CAD build for the part. Positions are in the model's coordinates, mm. Face numbers are marked on the shaded views. A direction names the side the tool comes from. Coordinates: 2 decimals unless noted, no trailing zeros. Order: outer loops, then holes, each group sorted by start corner. A loop starts at its lowest first (then second) coordinate and runs counter-clockwise, first axis right, second up. Notation, with made-up numbers: (88.5, 54) - (118.5, 54) arc R12 cw to (118.5, 63) - close; hole circle Ø7 at (-14.75, 31). An arc over 180 degrees is marked (long way). Use one line per item in the form item = value.
```python
from build123d import *

# Parameters (mm, degrees)
F0_R      = 8.89
F1_DEPTH  = 17.78
F2_R      = 7.747
F3_DEPTH  = 38.989
F4_R      = 8.89
F5_DEPTH  = 1.905
F6_R      = 7.747
F7_DEPTH  = 2.032
F8_R      = 8.89
F9_DEPTH  = 13.335
F10_R     = 7.747
F11_DEPTH = 2.032
F12_R     = 8.89
F13_DEPTH = 1.905
F14_R     = 7.747
F15_DEPTH = 12.7
F16_R     = 8.89
F17_DEPTH = 28.575
F18_R     = 6.477
F19_DEPTH = 27.559


with BuildPart() as f1:
    # F0 (on Right) → F1 (new body)
    with BuildSketch(Plane.YZ):
        Circle(F0_R)
    extrude(amount=F1_DEPTH)

    # F2 (on face) → F3 (join)
    with BuildSketch(Plane.YZ.offset(17.78)):
        Circle(F2_R)
    extrude(amount=F3_DEPTH)

    # F4 (on face) → F5 (join)
    with BuildSketch(Plane.YZ.offset(56.769)):
        Circle(F4_R)
    extrude(amount=F5_DEPTH)

    # F6 (on face) → F7 (join)
    with BuildSketch(Plane.YZ.offset(58.674)):
        Circle(F6_R)
    extrude(amount=F7_DEPTH)

    # F8 (on face) → F9 (join)
    with BuildSketch(Plane.YZ.offset(60.706)):
        Circle(F8_R)
    extrude(amount=F9_DEPTH)

    # F10 (on face) → F11 (join)
    with BuildSketch(Plane.YZ.offset(74.041)):
        Circle(F10_R)
    extrude(amount=F11_DEPTH)

    # F12 (on face) → F13 (join)
    with BuildSketch(Plane.YZ.offset(76.073)):
        Circle(F12_R)
    extrude(amount=F13_DEPTH)

    # F14 (on face) → F15 (join)
    with BuildSketch(Plane.YZ.offset(77.978)):
        Circle(F14_R)
    extrude(amount=F15_DEPTH)

    # F16 (on face) → F17 (join)
    with BuildSketch(Plane.YZ.offset(90.678)):
        Circle(F16_R)
    extrude(amount=F17_DEPTH)

    # F18 (on face) → F19 (cut)
    with BuildSketch(Plane.YZ.offset(119.253)):
        Circle(F18_R)
    extrude(amount=-F19_DEPTH, mode=Mode.SUBTRACT)


solid = f1.part
```
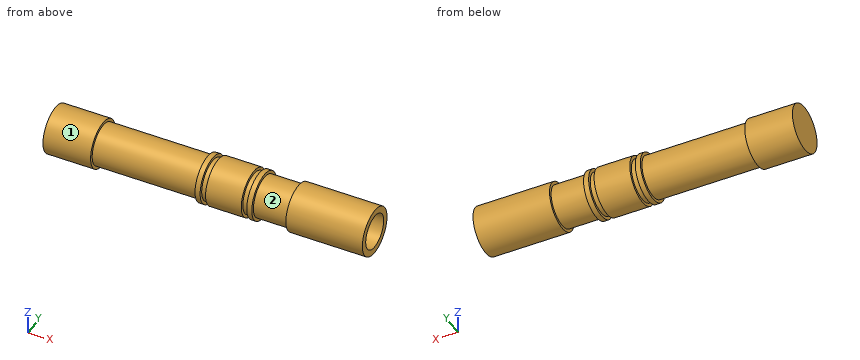
Item 1: Cut at B-B, the plane x = 36. Write the cut outline in (y, z), plus the area to 3 significant figures.
Derived:
outline = circle Ø15.49 at (0, 0)
area = 189 mm²
Item 2: 3-axis set-ups, long thin cutter, end or side, ignore diameter. For the marked faces 1 and 2: which of +Z, -Z, +X, -X, +Y, -Y reach the whole face in a straight line?
Derived:
face_1 = +X, -X
face_2 = none
Item 3: Cut at A-A, the plane x = 100. Write the cut outline in (y, z).
Derived:
outline = circle Ø17.78 at (0, 0); hole circle Ø12.95 at (0, 0)
Item 4: Drill centre lines: line 1 (X direction, y = 3.75, z = 8); line 2 (Z direction, x = 113, y = 0); line 3 (X direction, y = 0.75, z = 5.25). Where is each one in solid material? Low to high. Write a range as [from, to].
Derived:
line_1 = [0, 17.78], [56.77, 58.67], [60.71, 74.04], [76.07, 77.98], [90.68, 119.25]
line_2 = [-8.89, -6.48], [6.48, 8.89]
line_3 = [0, 91.69]
Item 5: Drop flat-ended pins along their axis: pin 1 (4 mm diameter, centred on y = 0, z = -1, fed in from +X); pin 2 (8 mm diameter, centred on x = 85, z = 4, fed in from -Y); pin 3 (5 mm diameter, centred on x = 86, y = -0.5, fed in from -Z). Give the stop position or say it passes through.
Derived:
pin_1 = 91.69
pin_2 = -7.75
pin_3 = -7.75
